from build123d import *

# Parameters (mm, degrees)
EXTRUDE007_DEPTH = 1.6
SKETCH004_W      = 114.99
SKETCH004_H      = 64.5
EXTRUDE006_DEPTH = 6
BOX_W            = 27
BOX_H            = 22
BOX_DEPTH        = 7
EXTRUDE_DEPTH    = 8.54
SKETCH003_R      = 2.5
EXTRUDE003_DEPTH = 3.6
SKETCH002_R      = 1.4
EXTRUDE004_DEPTH = 6


with BuildPart() as circuit_solid:
    # Sketch → Extrude007 (new body)
    with BuildSketch(Plane.XY):
        with BuildLine():
            Line((0, 1.02), (0, 63.48))
            ThreePointArc((1.02, 64.5), (0.298751, 64.201249), (0, 63.48))
            Line((1.02, 64.5), (133.97, 64.5))
            ThreePointArc((134.99, 63.48), (134.691249, 64.201249), (133.97, 64.5))
            Line((134.99, 63.48), (134.99, 45.7))
            Line((134.99, 45.7), (137.53, 43.16))
            Line((137.53, 43.16), (137.53, 9.96))
            Line((137.53, 9.96), (134.99, 7.42))
            Line((134.99, 7.42), (134.99, 1.02))
            ThreePointArc((133.97, 0), (134.691249, 0.298751), (134.99, 1.02))
            Line((133.97, 0), (1.02, 0))
            ThreePointArc((0, 1.02), (0.298751, 0.298751), (1.02, 0))
        make_face()
    extrude(amount=EXTRUDE007_DEPTH)


with BuildPart() as circuit_solid_1:
    # Extrude007 placement: moved
    add(circuit_solid.part.moved(Location((0, 0, 6.94))))


with BuildPart() as gap_solid:
    # Sketch004 → Extrude006 (new body)
    with BuildSketch(Plane.XY):
        with Locations((67.495, 32.25)):
            Rectangle(SKETCH004_W, SKETCH004_H)
    extrude(amount=EXTRUDE006_DEPTH)


with BuildPart() as gap_solid_1:
    # Extrude006 placement: moved
    add(gap_solid.part.moved(Location((0, 0, 2.54))))


with BuildPart() as gaps_solid:
    # Box → Box (new body)
    with BuildSketch(Plane(origin=(-4, 21.25, 2.54), x_dir=(1, 0, 0), z_dir=(0, 0, 1))):
        with Locations((13.5, 11)):
            Rectangle(BOX_W, BOX_H)
    extrude(amount=BOX_DEPTH)

    # Fusion: union circuit_solid, gap_solid
    add(circuit_solid_1.part)
    add(gap_solid_1.part)


with BuildPart() as shell:
    # Sketch001 → Extrude (new body)
    with BuildSketch(Plane.XY):
        with BuildLine():
            Line((1.02, 66.94), (133.97, 66.94))
            ThreePointArc((137.53, 63.38), (136.4873, 65.8973), (133.97, 66.94))
            Line((137.53, 63.38), (137.53, 1.02))
            ThreePointArc((133.97, -2.54), (136.4873, -1.4973), (137.53, 1.02))
            Line((133.97, -2.54), (1.02, -2.54))
            ThreePointArc((-2.54, 1.02), (-1.4973, -1.4973), (1.02, -2.54))
            Line((-2.54, 1.02), (-2.54, 63.38))
            ThreePointArc((1.02, 66.94), (-1.4973, 65.8973), (-2.54, 63.38))
        make_face()
    extrude(amount=EXTRUDE_DEPTH)

    # Cut: cut gaps_solid
    add(gaps_solid.part, mode=Mode.SUBTRACT)


with BuildPart() as sphere004:
    # Sphere004 → Sphere004 (revolve)
    with BuildSketch(Plane(origin=(96.52, 7.62, 0), x_dir=(1, 0, 0), z_dir=(0, -1, 0))):
        with BuildLine():
            ThreePointArc((0, -1.4), (1.4, 0), (0, 1.4))
            Line((0, 1.4), (0, -1.4))
        make_face()
    revolve(axis=Axis((96.52, 7.62, 0), (0, 0, 1)))


with BuildPart() as sphere005:
    # Sphere005 → Sphere005 (revolve)
    with BuildSketch(Plane(origin=(90.17, 55.88, 0), x_dir=(1, 0, 0), z_dir=(0, -1, 0))):
        with BuildLine():
            ThreePointArc((0, -1.4), (1.4, 0), (0, 1.4))
            Line((0, 1.4), (0, -1.4))
        make_face()
    revolve(axis=Axis((90.17, 55.88, 0), (0, 0, 1)))


with BuildPart() as sphere002:
    # Sphere002 → Sphere002 (revolve)
    with BuildSketch(Plane(origin=(66.04, 12.7, 0), x_dir=(1, 0, 0), z_dir=(0, -1, 0))):
        with BuildLine():
            ThreePointArc((0, -1.4), (1.4, 0), (0, 1.4))
            Line((0, 1.4), (0, -1.4))
        make_face()
    revolve(axis=Axis((66.04, 12.7, 0), (0, 0, 1)))


with BuildPart() as sphere001:
    # Sphere001 → Sphere001 (revolve)
    with BuildSketch(Plane(origin=(15.24, 55.88, 0), x_dir=(1, 0, 0), z_dir=(0, -1, 0))):
        with BuildLine():
            ThreePointArc((0, -1.4), (1.4, 0), (0, 1.4))
            Line((0, 1.4), (0, -1.4))
        make_face()
    revolve(axis=Axis((15.24, 55.88, 0), (0, 0, 1)))


with BuildPart() as sphere006:
    # Sphere006 → Sphere006 (revolve)
    with BuildSketch(Plane(origin=(128.27, 46.35, 0), x_dir=(1, 0, 0), z_dir=(0, -1, 0))):
        with BuildLine():
            ThreePointArc((0, -1.4), (1.4, 0), (0, 1.4))
            Line((0, 1.4), (0, -1.4))
        make_face()
    revolve(axis=Axis((128.27, 46.35, 0), (0, 0, 1)))


with BuildPart() as sphere003:
    # Sphere003 → Sphere003 (revolve)
    with BuildSketch(Plane(origin=(66.04, 40.64, 0), x_dir=(1, 0, 0), z_dir=(0, -1, 0))):
        with BuildLine():
            ThreePointArc((0, -1.4), (1.4, 0), (0, 1.4))
            Line((0, 1.4), (0, -1.4))
        make_face()
    revolve(axis=Axis((66.04, 40.64, 0), (0, 0, 1)))


with BuildPart() as pivot_top_solids:
    # Sphere → Sphere (revolve)
    with BuildSketch(Plane(origin=(13.97, 7.62, 0), x_dir=(1, 0, 0), z_dir=(0, -1, 0))):
        with BuildLine():
            ThreePointArc((0, -1.4), (1.4, 0), (0, 1.4))
            Line((0, 1.4), (0, -1.4))
        make_face()
    revolve(axis=Axis((13.97, 7.62, 0), (0, 0, 1)))

    # Fusion001: union Sphere004, Sphere005, Sphere002, Sphere001, Sphere006, Sphere003
    add(sphere004.part)
    add(sphere005.part)
    add(sphere002.part)
    add(sphere001.part)
    add(sphere006.part)
    add(sphere003.part)


with BuildPart() as pivot_top_solids_1:
    # Fusion001 placement: moved
    add(pivot_top_solids.part.moved(Location((0, 0, 8.54))))


with BuildPart() as pivot_base_solids:
    # Sketch003 → Extrude003 (new body)
    with BuildSketch(Plane.XY):
        with Locations((15.24, 55.88)):
            Circle(SKETCH003_R)
        with Locations((13.97, 7.62)):
            Circle(SKETCH003_R)
        with Locations((66.04, 40.64)):
            Circle(SKETCH003_R)
        with Locations((66.04, 12.7)):
            Circle(SKETCH003_R)
        with Locations((90.17, 55.88)):
            Circle(SKETCH003_R)
        with Locations((96.52, 7.62)):
            Circle(SKETCH003_R)
        with Locations((128.27, 46.35)):
            Circle(SKETCH003_R)
    extrude(amount=EXTRUDE003_DEPTH)


with BuildPart() as pivot_base_solids_1:
    # Extrude003 placement: moved
    add(pivot_base_solids.part.moved(Location((0, 0, 2.54))))


with BuildPart() as fusion003:
    # Sketch002 → Extrude004 (new body)
    with BuildSketch(Plane.XY):
        with Locations((15.24, 55.88)):
            Circle(SKETCH002_R)
        with Locations((13.97, 7.62)):
            Circle(SKETCH002_R)
        with Locations((66.04, 40.64)):
            Circle(SKETCH002_R)
        with Locations((66.04, 12.7)):
            Circle(SKETCH002_R)
        with Locations((90.17, 55.88)):
            Circle(SKETCH002_R)
        with Locations((96.52, 7.62)):
            Circle(SKETCH002_R)
        with Locations((128.27, 46.35)):
            Circle(SKETCH002_R)
    extrude(amount=EXTRUDE004_DEPTH)


with BuildPart() as fusion003_1:
    # Extrude004 placement: moved
    add(fusion003.part.moved(Location((0, 0, 2.54))))

    # Fusion002: union pivot_top_solids, pivot_base_solids
    add(pivot_top_solids_1.part)
    add(pivot_base_solids_1.part)


with BuildPart() as fusion003_2:
    # Fusion002 placement: moved
    add(fusion003_1.part.moved(Location((0.5, 0.5, 0))))

    # Fusion003: union shell
    add(shell.part)


solid = fusion003_2.part
Here's how the part is built. I have some questions about the finished solid (model axes, mm). A direction names the side the tool comes from. Coordinates: 2 decimals unless noted, no trailing zeros. Write each loop counter-clockwise with the first axis right and the second up, starting at its lowest first coordinate (ties: lowest second). Pieces come first, ordered by that corner, then holes.
Item 1: I want a section at B-B on y = 56.38. Write out the boundary of the cut face in (x, z).
Item 2: Will these pins go through, and if not, where does the flat tip stop? pin 1 (11 mm diameter, centred on x = 6.5, y = 9.5, fed in from +Z); pin 2 (1.5 mm diameter, centred on x = 15, y = 9, fed in from +Z); pin 3 (3 mm diameter, centred on y = 20, z = 8.5, fed in from +X).
Item 3: If we mould it in two halves opening along Y, with no side actions, what happens to faces 3 (the flat face through (73, -0.3, 8.54)), 4 (the cylindrical face through (-1.469, 65.925, 4.21)), 5 (the flat face through (67, 64.5, 5))? For each: +Y half, -Y half, draft (parallel to the pull), parting line (faces both ways), or undercut.
Item 4: I want a section at D-D on y = 37. Write out the boundary of the cut face in (x, z), and give its area (3 significant figures).
Item 5: I want a section at A-A on x = 128.77. Write out the boundary of the cut face in (y, z).
Item 6: I want a section at C-C on x = 80. Write out the boundary of the cut face in (y, z), and give its area (3 significant figures).
Item 7: If I drill on line 1 (X direction, y = 14.5, z = 5.25); line 2 (Y direction, x = 110, z = 3); line 3 (X direction, y = 58.5, z = 8), over which ranges is the centre line in solid material (lowest first)?
Item 8: On a 3-axis mill with a long thin cutter (end or side, diameter ignored), from which of +Z, -Z, +X, -X, +Y, -Y can I reach the whole of each face in a straight line? I mean faces 1 (the flat face through (136.28, 8.71, 7.73)), 2 (the flat face through (137.53, 33, 4)). Say none if no direction works.
Findings below:
1. outline: (-2.54, 0) - (137.53, 0) - (137.53, 8.54) - (134.99, 8.54) - (134.99, 6.94) - (124.99, 6.94) - (124.99, 2.54) - (93.17, 2.54) - (93.17, 6.14) - (92.07, 6.14) - (92.07, 8.54) arc R1.4 ccw to (89.27, 8.54) - (89.27, 6.14) - (88.17, 6.14) - (88.17, 2.54) - (18.24, 2.54) - (18.24, 6.14) - (17.14, 6.14) - (17.14, 8.54) arc R1.4 ccw to (14.34, 8.54) - (14.34, 6.14) - (13.24, 6.14) - (13.24, 2.54) - (10, 2.54) - (10, 6.94) - (0, 6.94) - (0, 8.54) - (-2.54, 8.54) - close
2. pin 1: stops at z = 6.94
2. pin 2: stops at z = 9.91
2. pin 3: stops at x = 0
3. face 3: draft
3. face 4: +Y half
3. face 5: undercut
4. outline: (-2.54, 0) - (137.53, 0) - (137.53, 6.94) - (124.99, 6.94) - (124.99, 2.54) - (-2.54, 2.54) - close
4. area: 411 mm2
5. outline: (-2.54, 0) - (66.94, 0) - (66.94, 8.54) - (64.5, 8.54) - (64.5, 6.94) - (48.25, 6.94) - (48.25, 8.54) arc R1.4 ccw to (45.45, 8.54) - (45.45, 6.94) - (0, 6.94) - (0, 8.54) - (-2.54, 8.54) - close
6. outline: (-2.54, 0) - (66.94, 0) - (66.94, 8.54) - (64.5, 8.54) - (64.5, 2.54) - (0, 2.54) - (0, 8.54) - (-2.54, 8.54) - close
6. area: 206 mm2
7. line 1: x = -2.54 to 10, 64.4 to 68.68, 124.99 to 137.53
7. line 2: y = -2.54 to 0, 64.5 to 66.94
7. line 3: x = -2.54 to 0, 134.99 to 137.53
8. face 1: +Z
8. face 2: +Z, -Z, +X, +Y, -Y
